Design review of the part shown in the three views and the two pictorial views. Dimensions are in mm from the part's minimum x, y and z. Round coordinates to 2 decimals unless told otherwise and drop trailing zeros. Loops run counter-clockwise (first coordinate to the right, second up) from the corner with the lowest first, then second, coordinate; pieces in that order, holes last. Notation, with made-up numbers: (89.5, 42.25) - (115.5, 42.25) arc R17 cw to (115.5, 69.25) - close; hole circle Ø3 at (7, 80). An arc over 180 degrees is marked (long way). Return JSON: item names as keys, results as strings. Group by question number.
(1) We need section D-D, the plane y = 5. Write out the cut boundary in (x, z).
(2) We need section C-C, the plane y = 0.5. Write out the cut boundary in (x, z), and give its area (3 significant figures).
(3) We need section B-B, the plane x = 2.75. Write out the cut boundary in (y, z).
(4) Wall thickness on L1, parallel to X at y = 1.2, z = 2.75; L2, parallel to Y at x = 1.7, z = 3.25: over which ranges is each line inside the solid? List them lowest first. Write a range as [from, to].
(5) We need section A-A, the plane z = 2.75. Write out the cut boundary in (x, y), and give its area (3 significant figures).
(6) The part is to be moulded in two halves that separate along Z. For the marked faces 1, 2 and 3, say which applies: pulls with the +Z half, pulls with the -Z half, needs draft (parallel to the pull), parting line crosses it, or undercut.
(7) Clearance check with flat-ended pins moving along their axes: pin 1 (1.9 mm diameter, centred on x = 3.5, z = 2.5, fed in from -Y); pin 2 (1.5 mm diameter, centred on y = 7.5, z = 4, fed in from -X). State where each tip first meets the part, or that it passes through.
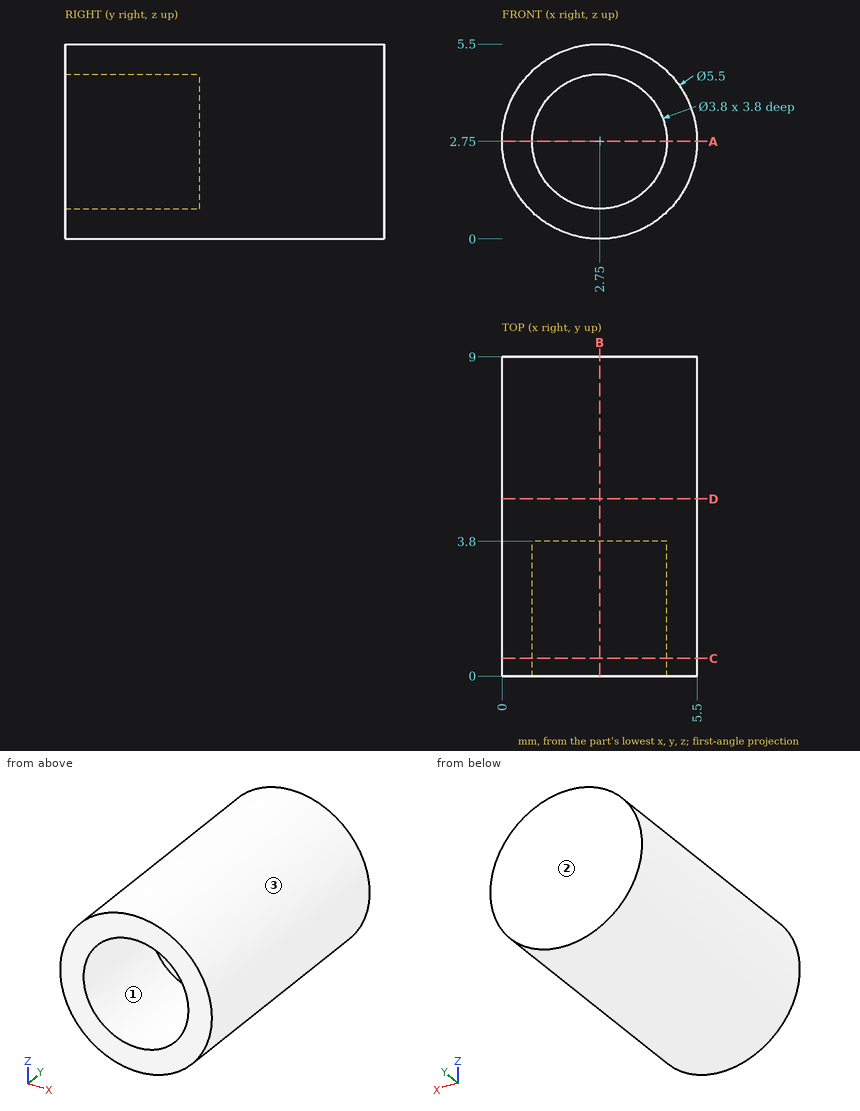
Solutions:
{
 "1": {"outline": "circle Ø5.5 at (2.75, 2.75)"},
 "2": {"outline": "circle Ø5.5 at (2.75, 2.75); hole circle Ø3.8 at (2.75, 2.75)", "area": "12.4 mm^2"},
 "3": {"outline": "(0, 0) - (9, 0) - (9, 5.5) - (0, 5.5) - (0, 4.65) - (3.8, 4.65) - (3.8, 0.85) - (0, 0.85) - close"},
 "4": {"L1": "[0, 0.85], [4.65, 5.5]", "L2": "[3.8, 9]"},
 "5": {"outline": "(0, 0) - (0.85, 0) - (0.85, 3.8) - (4.65, 3.8) - (4.65, 0) - (5.5, 0) - (5.5, 9) - (0, 9) - close", "area": "35.1 mm^2"},
 "6": {"face 1": "undercut", "face 2": "needs draft", "face 3": "parting line crosses it"},
 "7": {"pin 1": "y = 3.8", "pin 2": "x = 0.05"}
}
